For this review, take the finished solid that the model builds, in its own axes (mm). A direction names the side the tool comes from. Round coordinates to 2 decimals unless told otherwise and drop trailing zeros. Loops run counter-clockwise (first coordinate to the right, second up) from the corner with the lowest first, then second, coordinate; pieces in that order, holes last.
1) Take a section at B-B (z = 0). State the section outline as (x, y) points.
2) Take a section at C-C (y = -27). State the section outline as (x, z) points.
3) Tool access review of faces 4 (the cylindrical face through (-84.795, 19.594, 26.703)), 5 (the cylindrical face through (14.481, 3.042, 65.213)): name each direction out of +Z, -Z, +X, -X, +Y, -Y from which nothing blocks a thin tool from reaching the whole face with its end or side.
4) Wall thickness on L1, parallel to Z at x = 0, y = -20; L2, parallel to Z at x = 0, y = 1.25; L3, parallel to X at y = 3, z = -59.5: over which ranges is each line inside the solid? List them lowest first.
5) Insertion check: pin 1 (8 mm diameter, centred on y = 4.5, z = -12.5, fed in from +X); pin 2 (1.5 mm diameter, centred on y = -4, z = 45, fed in from +X); pin 3 (2 mm diameter, centred on x = 68.5, y = -6, fed in from -Z). Each pin has a flat end and moves straight along its axis. Give the tip position at first contact, or say it passes through.
6) Take a section at A-A (x = 0). State the section outline as (y, z) points.
7) Mouldability with a two-part tool opening along Z and no side actions: class faces 1 (the flat face through (-59, -31.384, -38)), 2 (the cylindrical face through (75.587, 0.277, 57.958)), 3 (the conical face through (-46.84, 13.56, 14.75)) as pulls with the +Z half, pulls with the -Z half, needs draft (parallel to the pull), parting line crosses it, or undercut.
Autodesk Inventor part; units mm, degrees
ref_plane "YZ Plane" through (0, 0, 0) normal (1, 0, 0) x (0, 1, 0)
ref_plane "XZ Plane" through (0, 0, 0) normal (0, 1, 0) x (-1, 0, 0)
ref_plane "XY Plane" through (0, 0, 0) normal (0, 0, 1) x (1, 0, 0)
sketch "Sketch1" plane through (0, 0, 0) normal (0, 0, 1) x (1, 0, 0)
  arc A0 (-28.9184, -1.6435) -> (-32.3684, 5.7551) centre (-35.052, 0) ccw
  line L0 (-28.702, 47.5942) -> (-28.702, -124.4009) construction
  line L1 (-32.3684, 5.7551) -> (-88.9, 32.1162)
  line L2 (-28.9184, -1.6435) -> (-86.2301, -215.5338)
  line L3 (-46.4564, 12.3244) -> (-66.802, 12.3244)
  line L4 (-60.4508, -95.6256) -> (-54.1008, -95.6256)
  line L5 (-73.152, -5.9838) -> (-73.152, -131.1779)
  line L6 (-73.152, -131.1779) -> (-63.627, -131.1779)
  line L7 (58.5667, 38.1) -> (-194.088, 38.1) construction
  line L8 (-95.25, 6.7162) -> (-95.25, -5.9838)
  line L9 (-95.25, 6.7162) -> (-88.9, 6.7162)
  line L10 (-88.9, 6.7162) -> (-88.9, 32.1162)
  line L11 (-95.25, -5.9838) -> (-73.152, -5.9838)
  line L12 (-95.25, -5.9838) -> (-95.25, -18.6838)
  line L13 (-95.25, -18.6838) -> (-89.3064, -18.6838)
  line L14 (-89.3064, -18.6838) -> (-89.3064, -24.6274)
  line L15 (-89.3064, -24.6274) -> (-95.25, -24.6274)
  line L16 (-95.25, -24.6274) -> (-95.25, -82.1838)
  line L17 (-95.25, -82.1838) -> (-82.55, -82.1838)
  line L18 (-89.3064, -18.6838) -> (-82.55, -18.6838)
  line L19 (-82.55, -18.6838) -> (-82.55, -82.1838)
  line L20 (-95.25, -82.1838) -> (-101.6, -82.1838)
  line L21 (-66.802, 12.3244) -> (-66.802, -31.3838)
  line L22 (-66.802, -31.3838) -> (-60.4508, -95.6256)
  line L23 (-82.55, -178.1009) -> (-76.2, -178.1009)
  line L24 (-82.55, -82.1838) -> (-82.55, -178.1009)
  line L25 (-86.2301, -215.5338) -> (-89.4051, -215.5338)
  line L26 (-89.4051, -215.5338) -> (-101.6, -82.1838)
  line L27 (-69.977, -5.9838) -> (-69.977, -31.3838)
  line L28 (-69.977, -31.3838) -> (-73.152, -31.3838)
  line L29 (-69.977, -5.9838) -> (-66.802, -5.9838)
  line L30 (-101.6, -82.1838) -> (-28.702, -82.1838) construction
  line L31 (0, -210.5351) -> (0, 86.485) construction
  point P0 (0, 0)
  dimension "d0" = 12.7
  dimension "d1" = 28.702
  dimension "d3" = 15
  dimension "d4" = 6.35
  dimension "d9" = 38.1
  dimension "d11" = 12.7
  dimension "d13" = 95.25
  dimension "d14" = 6.35
  dimension "d15" = 25.4
  dimension "d17" = 12.7
  dimension "d18" = 5.9436
  dimension "d19" = 5.9436
  dimension "d20" = 12.7
  dimension "d22" = 107.95
  dimension "d23" = 63.5
  dimension "d25" = 25.4
  dimension "d26" = 6.35
  dimension "d27" = 133.35
  dimension "d28" = 3.175
  dimension "d29" = 101.6
  dimension "d30" = 6.35
  dimension "d31" = 25
  dimension "d32" = 44.45
  dimension "d33" = 3.175
  dimension "d34" = 20.3456
  dimension "d35" = 9.525
revolve "Revolution1" add sketch "Sketch1" angle 360 about axis through (0, -210.5351, 0) along (0, 1, 0) contours L3 L21 L29 L27 L28 L5 L11 L8 L9 L10 L1
properties part number "phenolic_cap" material "Phenolic Resin"
Response:
1. outline: (-95.25, -5.98) - (-73.15, -5.98) - (-73.15, -31.38) - (-69.98, -31.38) - (-69.98, -5.98) - (-66.8, -5.98) - (-66.8, 12.32) - (-46.46, 12.32) - (-88.9, 32.12) - (-88.9, 6.72) - (-95.25, 6.72) - close; (46.46, 12.32) - (66.8, 12.32) - (66.8, -5.98) - (69.98, -5.98) - (69.98, -31.38) - (73.15, -31.38) - (73.15, -5.98) - (95.25, -5.98) - (95.25, 6.72) - (88.9, 6.72) - (88.9, 32.12) - close
2. outline: circle Ø146.3 at (0, 0); hole circle Ø139.95 at (0, 0)
3. face 4: +Y
3. face 5: -Y
4. L1: z = -73.15 to -69.98, 69.98 to 73.15
4. L2: z = -95.25 to -66.8, 66.8 to 95.25
4. L3: x = -74.38 to -30.37, 30.37 to 74.38
5. pin 1: stops at x = 94.87
5. pin 2: stops at x = 84.35
5. pin 3: stops at z = -67.2
6. outline: (-31.38, -73.15) - (-5.98, -73.15) - (-5.98, -95.25) - (6.72, -95.25) - (6.72, -88.9) - (32.12, -88.9) - (12.32, -46.46) - (12.32, -66.8) - (-5.98, -66.8) - (-5.98, -69.98) - (-31.38, -69.98) - close; (-31.38, 69.98) - (-5.98, 69.98) - (-5.98, 66.8) - (12.32, 66.8) - (12.32, 46.46) - (32.12, 88.9) - (6.72, 88.9) - (6.72, 95.25) - (-5.98, 95.25) - (-5.98, 73.15) - (-31.38, 73.15) - close
7. face 1: needs draft
7. face 2: parting line crosses it
7. face 3: undercut
